```python
from build123d import *

# Parameters (mm, degrees)
BOSS_EXTRUDE1_START = -8
SKETCH1_R           = 4
BOSS_EXTRUDE1_DEPTH = 38.1
SKETCH2_OUTSIDE_W   = 17.948
SKETCH2_OUTSIDE_H   = 48.048
CUT_EXTRUDE1_DEPTH  = 5
CUT_EXTRUDE2_DEPTH  = 30.290925305
SKETCH4_R           = 1.508332
CUT_EXTRUDE3_DEPTH  = 29.54645306
CUT_EXTRUDE4_DEPTH  = 1.216665


with BuildPart() as part:
    # Sketch1 → Boss-Extrude1 (new body)
    with BuildSketch(Plane(origin=(0, 0, 0), x_dir=(1, 0, 0), z_dir=(0, 1, 0)).offset(BOSS_EXTRUDE1_START)):
        with Locations(Location((0, 0, 0), (0, 0, 90))):
            Circle(SKETCH1_R)
    extrude(amount=BOSS_EXTRUDE1_DEPTH)

    # Sketch2 outside → Cut-Extrude1 (cut, symmetric)
    # profile 1 of 2: a face of its own
    with BuildSketch(Plane.XY):
        with Locations((0, 11.05)):
            Rectangle(SKETCH2_OUTSIDE_W, SKETCH2_OUTSIDE_H)
        with BuildLine():
            Line((-0.283333, -8), (-0.283333, 7.109115))
            ThreePointArc((-0.283333, 7.109115), (0.003787455, 7.935683585), (0.741491463, 8.406264691))
            ThreePointArc((0.741491463, 8.406264691), (2.828033272, 9.737268918), (3.64013247, 12.075157679))
            Line((3.64013247, 12.075157679), (3.64013247, 24.303947679))
            ThreePointArc((3.64013247, 24.303947679), (-0.04853801, 27.99261816), (-3.73720849, 24.303947679))
            Line((-3.73720849, 24.303947679), (-3.73720849, 8.666658))
            Line((-3.73720849, 8.666658), (-4, 8.666658))
            Line((-4, 8.666658), (-4, -8))
            Line((-4, -8), (-0.283333, -8))
        make_face(mode=Mode.SUBTRACT)
    # profile 2 of 2: a face of its own
    with BuildSketch(Plane.XY):
        with BuildLine():
            Line((2.38936199, 24.303947679), (2.38936199, 12.075157679))
            ThreePointArc((2.38936199, 12.075157679), (-0.04853801, 9.637257679), (-2.48643801, 12.075157679))
            Line((-2.48643801, 12.075157679), (-2.48643801, 24.303947679))
            ThreePointArc((-2.48643801, 24.303947679), (-0.04853801, 26.741847679), (2.38936199, 24.303947679))
        make_face()
    extrude(amount=CUT_EXTRUDE1_DEPTH, both=True, mode=Mode.SUBTRACT)

    # Sketch3 → Cut-Extrude2 (cut, through all)
    with BuildSketch(Plane(origin=(3.64013247, 0, 0), x_dir=(0, 0, -1), z_dir=(1, 0, 0))):
        with BuildLine():
            Line((-1.5, 6.333332), (-6.5, 6.333332))
            Line((-6.5, 6.333332), (-6.5, 36.333332))
            Line((-6.5, 36.333332), (0.5, 36.333332))
            Line((0.5, 36.333332), (0.5, 8.333332))
            ThreePointArc((0.5, 8.333332), (-0.085786438, 6.919118438), (-1.5, 6.333332))
        make_face()
        with BuildLine():
            Line((1.8, 36.333332), (1.8, 8.333332))
            ThreePointArc((1.8, 8.333332), (2.385786438, 6.919118438), (3.8, 6.333332))
            Line((3.8, 6.333332), (5.8, 6.333332))
            Line((5.8, 6.333332), (5.8, 36.333332))
            Line((5.8, 36.333332), (1.8, 36.333332))
        make_face()
    extrude(amount=-CUT_EXTRUDE2_DEPTH, mode=Mode.SUBTRACT)

    # Sketch4 → Cut-Extrude3 (cut, through all)
    with BuildSketch(Plane(origin=(-0.283333, 0, 0), x_dir=(0, 0, -1), z_dir=(1, 0, 0))):
        with Locations(Location((0, 0, 0), (0, 0, 90))):
            Circle(SKETCH4_R)
        with BuildLine():
            Line((-2.828427125, 0), (-2.828427125, -2))
            ThreePointArc((-2.828427125, -2), (0, -4.828427125), (2.828427125, -2))
            Line((2.828427125, -2), (2.828427125, 0))
            ThreePointArc((2.828427125, 0), (2.61312593, 1.0823922), (2, 2))
            Line((2, 2), (3.989952683, 3.989952683))
            Line((3.989952683, 3.989952683), (5, 3.989952683))
            Line((5, 3.989952683), (5, -11.010047317))
            Line((5, -11.010047317), (-5, -11.010047317))
            Line((-5, -11.010047317), (-5, 3.989952683))
            Line((-5, 3.989952683), (-3.989952683, 3.989952683))
            Line((-3.989952683, 3.989952683), (-2, 2))
            ThreePointArc((-2, 2), (-2.61312593, 1.0823922), (-2.828427125, 0))
        make_face()
    extrude(amount=-CUT_EXTRUDE3_DEPTH, mode=Mode.SUBTRACT)

    # Sketch5 → Cut-Extrude4 (cut)
    with BuildSketch(Plane(origin=(-0.283333, 0, 0), x_dir=(0, 0, -1), z_dir=(1, 0, 0))):
        with BuildLine():
            Line((-2.916664, 0), (-2.916664, -2.54))
            ThreePointArc((-2.916664, -2.54), (0, -5.456664), (2.916664, -2.54))
            Line((2.916664, -2.54), (2.916664, 0))
            ThreePointArc((2.916664, 0), (0, 2.916664), (-2.916664, 0))
        make_face()
    extrude(amount=-CUT_EXTRUDE4_DEPTH, mode=Mode.SUBTRACT)


solid = part.part
```
Geometry check sheet. Reference: the model listing, model coordinates, mm. A direction names the side the tool comes from. Give positions to 0.01 mm unless a question says otherwise; leave off trailing zeros. Write each loop counter-clockwise with the first axis right and the second up, starting at its lowest first coordinate (ties: lowest second). Pieces come first, ordered by that corner, then holes.
1) Section check A-A, the plane y = 20.5. Record the boundary of the cut face in (x, z), and give its area (3 significant figures).
2) Material ranges on L1, parallel to X at y = 3.5, z = -1.25; L2, parallel to X at y = -3, z = -0.5; L3, parallel to Z at x = -2.75, y = 19.5, recorded low to high.
3) Access from +Z, -Z, +X, -X, +Y, -Y to the whole of each face (thin tool, end or side, straight path). Record for faces 1 (the cylindrical face through (-2.25, 1.097, 2.607)), 2 (the cylindrical face through (-0.1, 26.74, -1.14)), 3 (the flat face through (-3, 18, -0.5)), 4 (the flat face through (3, 18, -1.8)).
4) Gauge pin test, flat ends, axial feed: pin 1 (4.5 mm diameter, centred on y = -0.5, z = 0, fed in from +X); pin 2 (1.2 mm diameter, centred on x = -2, z = 2.5, fed in from +Y); pin 3 (1.5 mm diameter, centred on y = 2, z = -2, fed in from +X). Record the tip position at first contact, or that the pin passes through.
5) Release check for a two-part mould opening along X. For faces 5 (the cylindrical face through (-0.113, 7.761, -1.165)), 6 (the flat face through (2.389, 18, -1)), 7 (the flat face through (-1, 3, -3)), 8 (the cylindrical face through (0.005, 9.638, -1.141)) record: pulls with the +X half, pulls with the -X half, needs draft (parallel to the pull), parting line crosses it, or undercut.
Computed:
1. outline: (-3.74, -1.43) arc R4 ccw to (-3.57, -1.8) - (-2.49, -1.8) - (-2.49, -0.5) - (-3.74, -0.5) - close; (2.39, -1.8) - (3.57, -1.8) arc R4 ccw to (3.64, -1.66) - (3.64, -0.5) - (2.39, -0.5) - close
1. area: 3.22 mm2
2. L1: x = -3.8 to -0.28
2. L2: x = -3.97 to -1.5
2. L3: z = -1.8 to -0.5
3. face 1: +Z, +X, -X
3. face 2: +Z, -Z
3. face 3: +Z, +X, -X, +Y
3. face 4: -Z, +X, -X, +Y
4. pin 1: stops at x = -1.5
4. pin 2: stops at y = 6.33
4. pin 3: stops at x = -0.28
5. face 5: pulls with the +X half
5. face 6: undercut
5. face 7: needs draft
5. face 8: undercut
